Model file for the job. Use its own axes, mm. A direction names the side the tool comes from. Round coordinates to 2 decimals unless told otherwise and drop trailing zeros. Loops run counter-clockwise (first coordinate to the right, second up) from the corner with the lowest first, then second, coordinate; pieces in that order, holes last. Notation, with made-up numbers: M 2,83.5 L 56,83.5 A20 ccw 56,87.5 Z; hole C 73,-13 d5. An arc over 180 degrees is marked long. Use a Markdown table: item, result. Add a question column.
Q1. Cut at A-A (y = 0). Give the cut face in (x, z).
Q2. Cut at D-D (y = -1.3). Give the cut face in (x, z).
Q3. Cut at C-C (x = 1.6). Give the cut face in (y, z), plus the area to 3 significant figures.
Q4. Cut at B-B (z = 28.5). Give the cut face in (x, y).
Q5. Pin check, flat tip, straight feed: pin 1 (1 mm diameter, centred on y = -0.5, z = 1.5, fed in from -X). Stop position of the tip, or through.
Q6. Tool access for faces 1 (the face through (0, 0, 0)), 2 (the face through (-1.2, 0, 3)), 3 (the face through (-1.5, 0, 30.4)): list every direction of +Z, -Z, +X, -X, +Y, -Y with a clear straight run to the whole face (end or side of a thin tool).
Q7. Probe line 1 (Z direction, x = -1.7, y = -0.1); line 2 (Y direction, x = -0.15, z = 14.5). List the from-to ranges inside material, lowest first. Write a range as from..to.
Autodesk Inventor part; units mm, degrees
ref_plane "YZ Plane" through (0, 0, 0) normal (1, 0, 0) x (0, 1, 0)
ref_plane "XZ Plane" through (0, 0, 0) normal (0, 1, 0) x (-1, 0, 0)
ref_plane "XY Plane" through (0, 0, 0) normal (0, 0, 1) x (1, 0, 0)
sketch "スケッチ1" plane through (0, 0, 0) normal (0, 0, 1) x (1, 0, 0)
  circle A0 centre (0, 0) radius 2
  dimension "d0" = 4
extrude "押し出し1" add sketch "スケッチ1" along normal blind 36.4
sketch "スケッチ2" plane through (0, 0, 36.4) normal (0, 0, 1) x (1, 0, 0)
  circle A0 centre (0, 0) radius 2
  line L0 (-1.2, -1.6) -> (-1.2, 1.6)
  circle A1 centre (0, 0) radius 2
  dimension "d4" = 3.2
extrude "押し出し2" cut sketch "スケッチ2" against normal blind 6 contours L0 A0 picked at (-1.3118, -0.4272)
sketch "スケッチ3" plane through (0, 0, 0) normal (0, 0, -1) x (-1, 0, 0)
  line L0 (1.2, 1.6) -> (1.2, -1.6)
  circle A0 centre (0, 0) radius 2
  dimension "d7" = 3.2
extrude "押し出し3" cut sketch "スケッチ3" against normal blind 6 contours A0 L0 picked at (1.6903, 0)
properties part number "shaft" material "アルミニウム 5052 H32"
Checked values:
| question | item | result |
|---|---|---|
| 1 | outline | M -2,6 L -1.2,6 L -1.2,0 L 2,0 L 2,36.4 L -1.2,36.4 L -1.2,30.4 L -2,30.4 Z |
| 2 | outline | M -1.52,6 L -1.2,6 L -1.2,0 L 1.52,0 L 1.52,36.4 L -1.2,36.4 L -1.2,30.4 L -1.52,30.4 Z |
| 3 | outline | M -1.2,0 L 1.2,0 L 1.2,36.4 L -1.2,36.4 Z |
| 3 | area | 87.4 mm^2 |
| 4 | outline | C 0,0 d4 |
| 5 | pin 1 | stops at x = -1.2 |
| 6 | face 1 | -Z, +X, -X, +Y, -Y |
| 6 | face 2 | -Z, -X, +Y, -Y |
| 6 | face 3 | +Z, -X, +Y, -Y |
| 7 | line 1 | z = 6..30.4 |
| 7 | line 2 | y = -1.99..1.99 |
